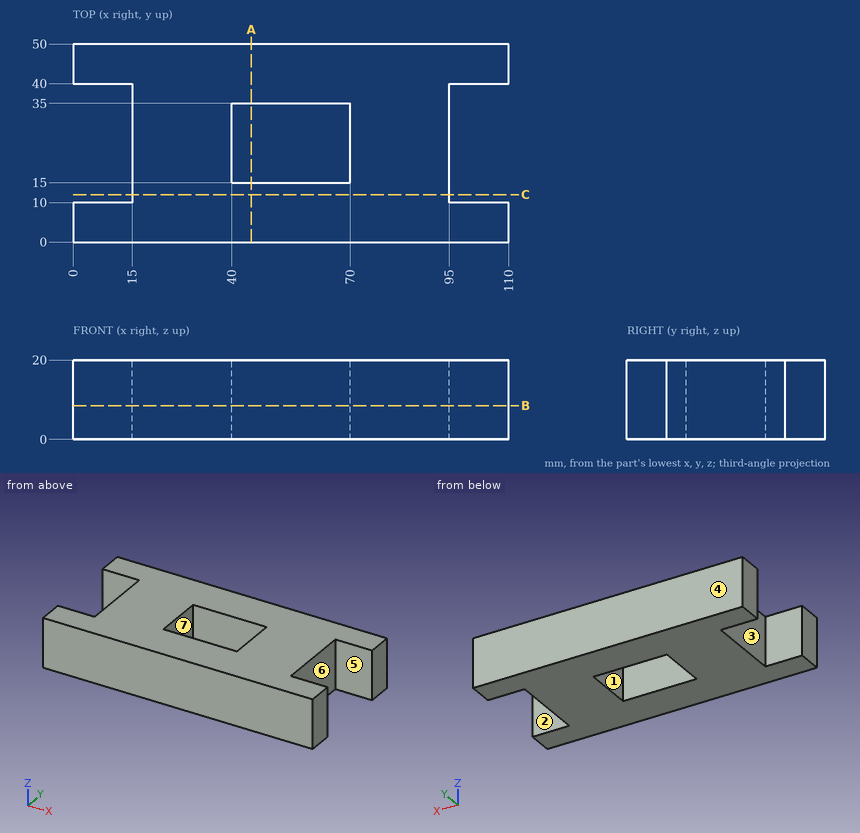
Study the drawing (mm; zero at the part's minimum x, y, z) and answer. A direction names the side the tool comes from. Give positions to 0.01 mm unless a question says otherwise; leave off trailing zeros. Loops run counter-clockwise (first coordinate to the right, second up) from the corner with the lowest first, then second, coordinate; pieces in that order, holes last. Notation, with made-up numbers: (11, 37.25) - (22, 37.25) arc R22 cw to (22, 70.25) - close; hole circle Ø8 at (3.25, 35). An arc over 180 degrees is marked (long way). Answer in a Markdown table with one row per item. Add a question column.
Q1. Each of these flat-tipped pins is pushed along its axis until it touches: P1, Ø4, axis at y = 14, z = 8.5, coming from the -X side; P2, Ø10, axis at y = 26.5, z = 14, coming from the +X side. Where does it stop, or does it pass through?
Q2. Consider line 1 along Y through (x, z) = (103.5, 15.5); line 2 along Y through (x, z) = (42, 2); line 3 along X through (y, z) = (24, 14). Determine where each line is inside the solid, lowest interval first.
Q3. The part is cut by section C-C (y = 12). Determine the outline of the cut face in (x, z), and give its area (3 significant figures).
Q4. The part is cut by section B-B (z = 8.5). Determine the outline of the cut face in (x, y), and give its area (3 significant figures).
Q5. The part is cut by section A-A (x = 45). Determine the outline of the cut face in (y, z).
Q6. Determine the mould class of the marked faces 5, 6 and 7 for opening direction X: released by +X, released by -X, zero draft, split by the parting line, or undercut.
Q7. A tool of negligible diameter and unlimited length cuts with its end or side. For the marked faces 1, 2, 3 and 4, from which of +Z, -Z, +X, -X, +Y, -Y can it reach the whole face along a straight path? Write none if from no direction.
Solution:
| question | item | result |
|---|---|---|
| 1 | P1 | stops at x = 15 |
| 1 | P2 | stops at x = 95 |
| 2 | line 1 | y = 0 to 10, 40 to 50 |
| 2 | line 2 | y = 0 to 15, 35 to 50 |
| 2 | line 3 | x = 15 to 40, 70 to 95 |
| 3 | outline | (15, 0) - (95, 0) - (95, 20) - (15, 20) - close |
| 3 | area | 1,600 mm² |
| 4 | outline | (0, 0) - (110, 0) - (110, 10) - (95, 10) - (95, 40) - (110, 40) - (110, 50) - (0, 50) - (0, 40) - (15, 40) - (15, 10) - (0, 10) - close; hole (40, 15) - (70, 15) - (70, 35) - (40, 35) - close |
| 4 | area | 4,000 mm² |
| 5 | outline | (0, 0) - (15, 0) - (15, 20) - (0, 20) - close; (35, 0) - (50, 0) - (50, 20) - (35, 20) - close |
| 6 | face 5 | zero draft |
| 6 | face 6 | released by +X |
| 6 | face 7 | undercut |
| 7 | face 1 | +Z, -Z |
| 7 | face 2 | +Z, -Z, +X |
| 7 | face 3 | +Z, -Z, -X |
| 7 | face 4 | +Z, -Z, +X, -X, +Y |
